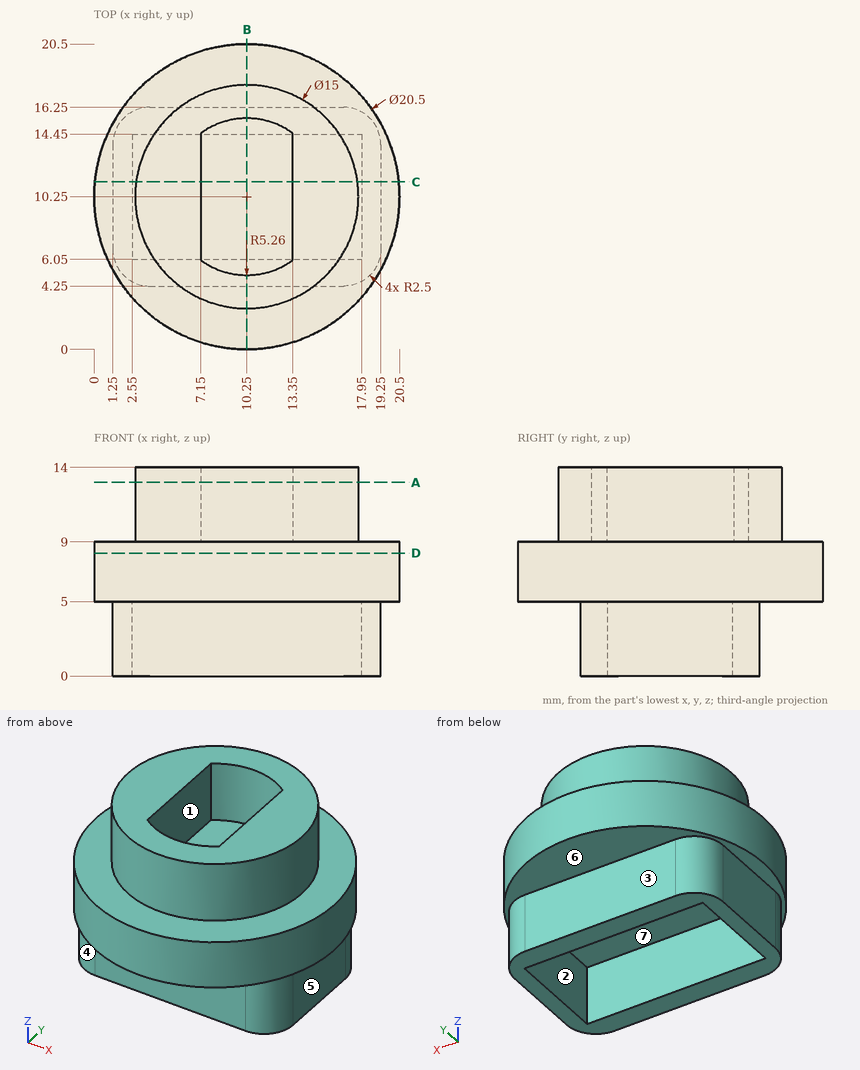
Print and shaded views of the part. All mm, measured from the part's lowest x, y and z. A direction names the side the tool comes from. Coordinates: 2 decimals unless noted, no trailing zeros. Order: outer loops, then holes, each group sorted by start corner. A loop starts at its lowest first (then second) coordinate and runs counter-clockwise, first axis right, second up.
(1) Slice it at A-A, the plane z = 13. Write the cut outline in (x, y).
Check sheet entries:
outline: circle Ø15 at (10.25, 10.25); hole (7.15, 6) arc R5.26 ccw to (13.35, 6) - (13.35, 14.5) arc R5.26 ccw to (7.15, 14.5) - close
(2) Tool access for the marked faces 1, 2, 3 and 4: list every direction of +Z, -Z, +X, -X, +Y, -Y with a clear straight run to the whole face (end or side of a thin tool).
Check sheet entries:
face 1: +Z
face 2: -Z
face 3: -Z, +X, -X, +Y
face 4: -Z, -X, -Y
(3) Probe L1, parallel to Y at x = 14, z = 4.25; L2, parallel to X at y = 6.75, z = 1.5; L3, parallel to Z at x = 11.5, y = 14.5. List the from-to ranges inside material, lowest first.
Check sheet entries:
L1: y = 4.25 to 6.05, 14.45 to 16.25
L2: x = 1.25 to 2.55, 17.95 to 19.25
L3: z = 0 to 9
(4) Pin check, flat tips, straight feed: pin 1 Ø1 at (y, z) = (17, 11) entering from +X (1 decimal); pin 2 Ø3 at (y, z) = (13, 7.5) entering from +X; pin 3 Ø8 at (y, z) = (8.5, 6) entering from -X; pin 4 Ø5.5 at (y, z) = (8.5, 11.5) entering from +X. Stop position of each tip, or through.
Check sheet entries:
pin 1: stops at x = 14.4
pin 2: stops at x = 20.42
pin 3: stops at x = 0
pin 4: stops at x = 20.48
(5) Slice it at D-D, the plane z = 8.25. Write the cut outline in (x, y), and give its area (3 significant figures).
Check sheet entries:
outline: circle Ø20.5 at (10.25, 10.25)
area: 330 mm2
(6) Slice it at B-B, the plane x = 10.25. Write the cut outline in (y, z), and give its area (3 significant figures).
Check sheet entries:
outline: (0, 5) - (4.25, 5) - (4.25, 0) - (6.05, 0) - (6.05, 5) - (14.45, 5) - (14.45, 0) - (16.25, 0) - (16.25, 5) - (20.5, 5) - (20.5, 9) - (17.75, 9) - (17.75, 14) - (15.51, 14) - (15.51, 9) - (4.99, 9) - (4.99, 14) - (2.75, 14) - (2.75, 9) - (0, 9) - close
area: 122 mm2
(7) Pull direction X, two halves, no side cores. Call the marked faces 5, 6 and 7: pulls with the +X half, pulls with the -X half, needs draft (parallel to the pull), parting line crosses it, or undercut.
Check sheet entries:
face 5: pulls with the +X half
face 6: needs draft
face 7: undercut
(8) Slice it at C-C, the plane y = 11.25. Write the cut outline in (x, z), and give its area (3 significant figures).
Check sheet entries:
outline: (0.05, 5) - (1.25, 5) - (1.25, 0) - (2.55, 0) - (2.55, 5) - (17.95, 5) - (17.95, 0) - (19.25, 0) - (19.25, 5) - (20.45, 5) - (20.45, 9) - (17.68, 9) - (17.68, 14) - (13.35, 14) - (13.35, 9) - (7.15, 9) - (7.15, 14) - (2.82, 14) - (2.82, 9) - (0.05, 9) - close
area: 138 mm2
